from build123d import *

# Parameters (mm, degrees)
SKETCH1_W           = 70
SKETCH1_H           = 40
BOSS_EXTRUDE1_DEPTH = 30
CUT_EXTRUDE1_DEPTH  = 41
CUT_EXTRUDE2_DEPTH  = 31
SKETCH4_W           = 15
SKETCH4_H           = 4.024531718
CUT_EXTRUDE3_DEPTH  = 71
SKETCH5_R           = 5
CUT_EXTRUDE4_DEPTH  = 41


with BuildPart() as part:
    # Sketch1 → Boss-Extrude1 (new body)
    with BuildSketch(Plane(origin=(0, 0, 0), x_dir=(1, 0, 0), z_dir=(0, 1, 0))):
        with Locations((35, 20)):
            Rectangle(SKETCH1_W, SKETCH1_H)
    extrude(amount=BOSS_EXTRUDE1_DEPTH)

    # Sketch2 → Cut-Extrude1 (cut, through all)
    with BuildSketch(Plane.XY):
        Polygon((70, 30), (30, 30), (70, 10), align=None)
    extrude(amount=-CUT_EXTRUDE1_DEPTH, mode=Mode.SUBTRACT)

    # Sketch3 → Cut-Extrude2 (cut, through all)
    with BuildSketch(Plane(origin=(0, 0, 0), x_dir=(-1, 0, 0), z_dir=(0, -1, 0))):
        Polygon((-70, 0), (-45, 0), (-70, 20), align=None)
    extrude(amount=-CUT_EXTRUDE2_DEPTH, mode=Mode.SUBTRACT)

    # Sketch4 → Cut-Extrude3 (cut, through all)
    with BuildSketch(Plane.ZY):
        with Locations((-22.5, 27.987734141)):
            Rectangle(SKETCH4_W, SKETCH4_H)
    extrude(amount=-CUT_EXTRUDE3_DEPTH, mode=Mode.SUBTRACT)

    # Sketch5 → Cut-Extrude4 (cut, through all)
    with BuildSketch(Plane.XY):
        with Locations((15, 15)):
            Circle(SKETCH5_R)
    extrude(amount=-CUT_EXTRUDE4_DEPTH, mode=Mode.SUBTRACT)


solid = part.part
Work out the finished part from the listing and answer in its coordinate system (mm). A direction names the side the tool comes from. Coordinates: 2 decimals unless noted, no trailing zeros. Loops run counter-clockwise (first coordinate to the right, second up) from the corner with the lowest first, then second, coordinate; pieces in that order, holes last. Notation, with made-up numbers: (87, -21) -> (103, -21) arc R35 ccw to (103, 13) -> close; hole circle Ø4 at (-5.5, 63.25). An arc over 180 degrees is marked (long way). Write each question's results on one line, items separated by ' | '. Start each with the question number.
1) Find section C-C on x = 6.5. Determine the outline of the cut face in (y, z).
2) For faces 1 (the cylindrical face through (17.307, 10.564, -19.72)), 2 (the flat face through (19, 28, -30)), determine the directions among +Z, -Z, +X, -X, +Y, -Y from which every point of the face is accessible in a straight line to the end or side of a thin tool.
3) Find section A-A on y = 27.25. Determine the outline of the cut face in (x, z).
4) Find section D-D on y = 5.75. Determine the outline of the cut face in (x, z).
5) Find section B-B on x = 15. Determine the outline of the cut face in (y, z).
6) Flat-ended cylindrical pins translate along their axes: P1, Ø4.5, axis at x = 17, y = 27, coming from the +Z side; P2, Ø6, axis at y = 18.5, z = -35.5, coming from the +X side; P3, Ø5, axis at x = 42, z = -7, coming from the +Y side; P4, Ø5, axis at x = 34.5, z = -18, coming from the +Y side. Find the tip coordinate at first contact, or state that the pin passes through.
7) Consider line 1 along Z through (x, y) = (26, 26.25); line 2 along Y through (x, z) = (15, -29.5); line 3 along Y through (x, z) = (15, -13.5). Determine where each line is inside the solid, lowest interval first.
8) The mould has two halves that part along Z. Classify faces 3 (the flat face through (27, 11, -40)), 4 (the flat face through (22, 15, 0)), 5 (the flat face through (19, 25.975, -23)), 6 (the flat face through (70, 5, -30)): pulls with the +Z half, pulls with the -Z half, needs draft (parallel to the pull), parting line crosses it, or undercut.
Response values:
1) outline: (0, -40) -> (30, -40) -> (30, -30) -> (25.98, -30) -> (25.98, -15) -> (30, -15) -> (30, 0) -> (0, 0) -> close
2) face 1: +Z, -Z | face 2: +X, -X, +Y
3) outline: (0, -40) -> (35.5, -40) -> (35.5, -30) -> (0, -30) -> close; (0, -15) -> (35.5, -15) -> (35.5, 0) -> (0, 0) -> close
4) outline: (0, -40) -> (70, -40) -> (70, -20) -> (45, 0) -> (0, 0) -> close
5) outline: (0, -40) -> (10, -40) -> (10, 0) -> (0, 0) -> close; (20, -40) -> (30, -40) -> (30, -30) -> (25.98, -30) -> (25.98, -15) -> (30, -15) -> (30, 0) -> (20, 0) -> close
6) P1: stops at z = 0 | P2: stops at x = 59 | P3: stops at y = 25.25 | P4: stops at y = 25.98
7) line 1: z = -40 to -30, -15 to 0 | line 2: y = 0 to 10, 20 to 25.98 | line 3: y = 0 to 10, 20 to 30
8) face 3: pulls with the -Z half | face 4: pulls with the +Z half | face 5: undercut | face 6: needs draft
